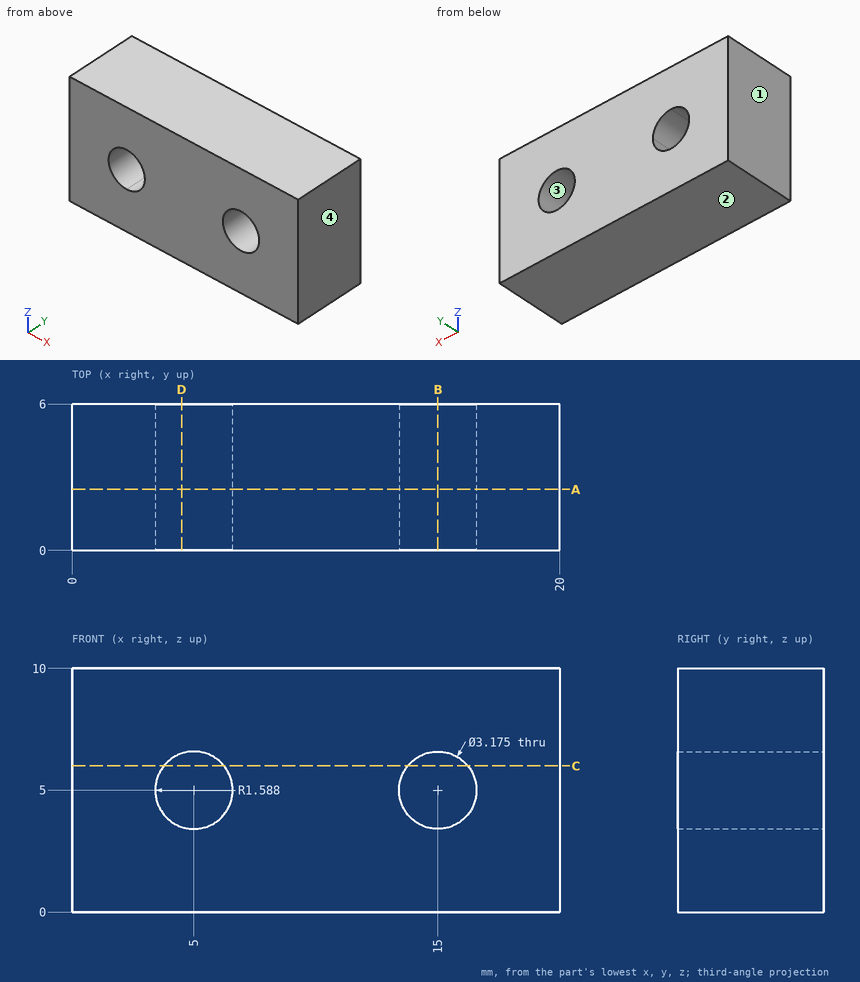
The figure shows three views and two pictorial views of one solid part (mm, origin at its lowest corner). Answer the questions. Coordinates: 2 decimals unless noted, no trailing zeros. Write each loop counter-clockwise with the first axis right and the second up, starting at its lowest first coordinate (ties: lowest second). Pieces come first, ordered by that corner, then holes. Notation, with made-up numbers: (-26, 21.5) -> (-12, 21.5) arc R24 ccw to (-12, 54.5) -> close; hole circle Ø5 at (78, 82). An arc over 180 degrees is marked (long way). Return JSON: item names as keys, results as strings.
1. A cutting plane is placed at C-C (z = 6). Determine the outline of the cut face in (x, y).
Found:
{"outline": "(0, 0) -> (3.77, 0) -> (3.77, 6) -> (0, 6) -> close; (6.23, 0) -> (13.77, 0) -> (13.77, 6) -> (6.23, 6) -> close; (16.23, 0) -> (20, 0) -> (20, 6) -> (16.23, 6) -> close"}
2. A cutting plane is placed at B-B (x = 15). Determine the outline of the cut face in (y, z).
Found:
{"outline": "(0, 0) -> (6, 0) -> (6, 3.41) -> (0, 3.41) -> close; (0, 6.59) -> (6, 6.59) -> (6, 10) -> (0, 10) -> close"}
3. Find the intervals of material crossed by line 1 along X through (y, z) = (1.9, 5); line 2 along X through (y, z) = (3.45, 4.25); line 3 along Z through (x, y) = (15.25, 1.1), in increasing order. Write a range as from..to.
Found:
{"line 1": "0..3.41, 6.59..13.41, 16.59..20", "line 2": "0..3.6, 6.4..13.6, 16.4..20", "line 3": "0..3.43, 6.57..10"}
4. A cutting plane is placed at D-D (x = 4.5). Determine the outline of the cut face in (y, z).
Found:
{"outline": "(0, 0) -> (6, 0) -> (6, 3.49) -> (0, 3.49) -> close; (0, 6.51) -> (6, 6.51) -> (6, 10) -> (0, 10) -> close"}
5. Determine the mould class of the marked faces 1, 2, 3 and 4 for opening direction X: pulls with the +X half, pulls with the -X half, needs draft (parallel to the pull), parting line crosses it, or undercut.
Found:
{"face 1": "pulls with the -X half", "face 2": "needs draft", "face 3": "undercut", "face 4": "pulls with the +X half"}
6. A cutting plane is placed at A-A (y = 2.5). Determine the outline of the cut face in (x, z) (1 decimal), and give its area (3 significant figures).
Found:
{"outline": "(0, 0) -> (20, 0) -> (20, 10) -> (0, 10) -> close; hole circle Ø3.2 at (5, 5); hole circle Ø3.2 at (15, 5)", "area": "184 mm2"}
